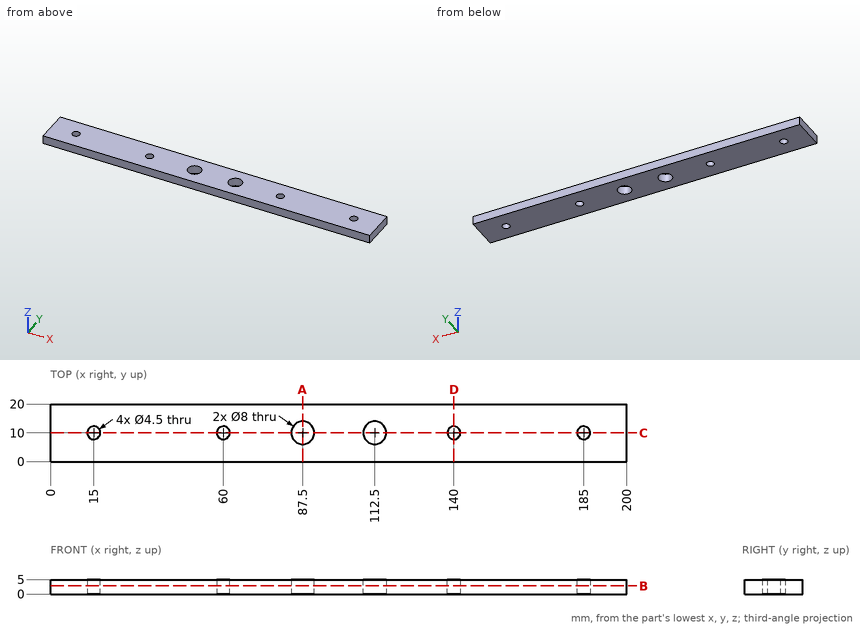
Source: three-view drawing plus pictorial views. Frame: mm from the lowest corner of the part. Round coordinates to 2 decimals unless told otherwise and drop trailing zeros. Order: outer loops, then holes, each group sorted by start corner. A loop starts at its lowest first (then second) coordinate and runs counter-clockwise, first axis right, second up. Notation, with made-up numbers: M 34,24.5 L 91,24.5 A14 cw 91,39.5 Z; hole C 47,26.5 d8. An arc over 180 degrees is marked long. One line per item, written item: value.
(1) Cut plane D-D (x = 140). Return the cut outline in (y, z), and give its area (3 significant figures).
Result sheet:
outline: M 0,0 L 7.75,0 L 7.75,5 L 0,5 Z; M 12.25,0 L 20,0 L 20,5 L 12.25,5 Z
area: 77.5 mm2
(2) Line query: probe 1 along Y at (x, z) = (15, 1.8); probe 2 along Y at (x, z) = (87.5, 3.15). Output: solid intervals per line, ascending. Write a range as [from, to].
Result sheet:
probe 1: [0, 7.75], [12.25, 20]
probe 2: [0, 6], [14, 20]
(3) Cut plane B-B (z = 2.85). Return the cut outline in (x, y).
Result sheet:
outline: M 0,0 L 200,0 L 200,20 L 0,20 Z; hole C 15,10 d4.5; hole C 60,10 d4.5; hole C 87.5,10 d8; hole C 112.5,10 d8; hole C 140,10 d4.5; hole C 185,10 d4.5
(4) Cut plane A-A (x = 87.5). Return the cut outline in (y, z), and give its area (3 significant figures).
Result sheet:
outline: M 0,0 L 6,0 L 6,5 L 0,5 Z; M 14,0 L 20,0 L 20,5 L 14,5 Z
area: 60.0 mm2
(5) Pin query (flat end, axial travel): P1, Ø7, axis at x = 112.5, y = 10, coming from the +Z side. Return the tip coordinate at first contact, or that it passes through.
Result sheet:
P1: through
(6) Cut plane C-C (y = 10). Return the cut outline in (x, z).
Result sheet:
outline: M 0,0 L 12.75,0 L 12.75,5 L 0,5 Z; M 17.25,0 L 57.75,0 L 57.75,5 L 17.25,5 Z; M 62.25,0 L 83.5,0 L 83.5,5 L 62.25,5 Z; M 91.5,0 L 108.5,0 L 108.5,5 L 91.5,5 Z; M 116.5,0 L 137.75,0 L 137.75,5 L 116.5,5 Z; M 142.25,0 L 182.75,0 L 182.75,5 L 142.25,5 Z; M 187.25,0 L 200,0 L 200,5 L 187.25,5 Z
